Could you check a few things on this model? Use its own coordinates, in mm. Round coordinates to 2 decimals unless told otherwise and drop trailing zeros. Order: outer loops, then holes, each group sorted by start corner. A loop starts at its lowest first (then second) coordinate and runs counter-clockwise, first axis right, second up.
```python
from build123d import *

# Parameters (mm, degrees)
SKETCH1_W                                = 73
SKETCH1_H                                = 48
BOSS_EXTRUDE1_DEPTH                      = 1.6
CUT_EXTRUDE1_DEPTH                       = 44.712812767
MIRROR1_AT_THE_SECOND_PLANE_COPY_1_DEPTH = 44.712812767
FILLET1_R                                = 2
SKETCH3_R                                = 1.5
CUT_EXTRUDE2_DEPTH                       = 44.712812767


with BuildPart() as part:
    # Sketch1 → Boss-Extrude1 (new body)
    with BuildSketch(Plane.XY):
        Rectangle(SKETCH1_W, SKETCH1_H)
    extrude(amount=BOSS_EXTRUDE1_DEPTH)

    # Sketch2 → Cut-Extrude1 (cut, through all)
    with BuildSketch(Plane.XY.offset(1.6)):
        with BuildLine():
            Line((-27.5, 23), (-27.5, 24))
            Line((-27.5, 24), (-36.5, 24))
            Line((-36.5, 24), (-36.5, 15))
            Line((-36.5, 15), (-35.5, 15))
            ThreePointArc((-35.5, 15), (-29.843145751, 17.343145751), (-27.5, 23))
        make_face()
    cut_extrude1 = extrude(amount=-CUT_EXTRUDE1_DEPTH, mode=Mode.SUBTRACT)

    # Mirror1: Cut-Extrude1 across plane
    add(cut_extrude1.mirror(Plane(origin=(0, 0, 0), x_dir=(0, 0, 1), z_dir=(1, 0, 0))), mode=Mode.SUBTRACT)

    # Mirror1 at the second plane: Cut-Extrude1 across plane
    add(cut_extrude1.mirror(Plane.ZX), mode=Mode.SUBTRACT)

    # Mirror1 at the second plane copy 1 sketc → Mirror1 at the second plane copy 1 (cut, through all)
    with BuildSketch(Plane(origin=(0, 0, 1.6), x_dir=(-1, 0, 0), z_dir=(0, 0, 1))):
        with BuildLine():
            Line((-27.5, 23), (-27.5, 24))
            Line((-27.5, 24), (-36.5, 24))
            Line((-36.5, 24), (-36.5, 15))
            Line((-36.5, 15), (-35.5, 15))
            ThreePointArc((-35.5, 15), (-29.843145751, 17.343145751), (-27.5, 23))
        make_face()
    extrude(amount=-MIRROR1_AT_THE_SECOND_PLANE_COPY_1_DEPTH, mode=Mode.SUBTRACT)

    # Fillet1
    # the kernel refuses this fillet: 2 mm, written as the material it takes off along each edge
    with BuildSketch(Plane(origin=(-36.5, 15, 6.474685928), x_dir=(0.9997519364152339, 0.022272530929157337, 0), z_dir=(0, 0, -1)), Plane(origin=(-27.5, -24, 6.474685928), x_dir=(-0.022272530929167148, 0.9997519364152335, 0), z_dir=(0, 0, -1)), Plane(origin=(36.5, -15, 6.474685928), x_dir=(-0.9997519364152339, -0.022272530929157337, 0), z_dir=(0, 0, -1))) as fillet1_piece_1:
        with BuildLine():
            CenterArc((1.956075236, 1.99393574), FILLET1_R, 181.276227552, 84.260829523)
            Line((-0.043428637, 1.949390678), (-0.243379025, 1.944936172))
            Line((-0.243379025, 1.944936172), (-0.199950387, -0.004454506))
            Line((-0.199950387, -0.004454506), (0.004454506, -0.199950387))
            ThreePointArc((0.004454506, -0.199950387), (1.004206443, -0.177677856), (1.784883764, -0.199393574))
            Line((1.784883764, -0.199393574), (1.800446625, 0))
        make_face()
    extrude(amount=11.349371855, mode=Mode.SUBTRACT)
    with BuildSketch(Plane(origin=(-27.5, 24, 6.474685928), x_dir=(1, 0, 0), z_dir=(0, 0, -1)), Plane(origin=(-36.5, -15, 6.474685928), x_dir=(0, 1, 0), z_dir=(0, 0, -1)), Plane(origin=(36.5, 15, 6.474685928), x_dir=(0, -1, 0), z_dir=(0, 0, -1)), Plane(origin=(27.5, -24, 6.474685928), x_dir=(-1, 0, 0), z_dir=(0, 0, -1))) as fillet1_piece_2:
        with BuildLine():
            CenterArc((1.949874371, 2), FILLET1_R, 185.739170477, 84.260829523)
            Line((-0.040100503, 1.8), (-0.239097991, 1.78))
            ThreePointArc((-0.239097991, 1.78), (-0.2, 1), (-0.2, 0))
            Line((-0.2, 0), (0, -0.2))
            Line((0, -0.2), (1.949874371, -0.2))
            Line((1.949874371, -0.2), (1.949874371, 0))
        make_face()
    extrude(amount=11.349371855, mode=Mode.SUBTRACT)
    with BuildSketch(Plane(origin=(27.5, 24, 6.474685928), x_dir=(-1, 0, 0), z_dir=(0, 0, -1))) as fillet1_piece_3:
        with BuildLine():
            CenterArc((1.949874371, -2), FILLET1_R, 90, 84.260829523)
            Line((-0.040100503, -1.8), (-0.239097991, -1.78))
            ThreePointArc((-0.239097991, -1.78), (-0.2, -1), (-0.2, 0))
            Line((-0.2, 0), (0, 0.2))
            Line((0, 0.2), (1.949874371, 0.2))
            Line((1.949874371, 0.2), (1.949874371, 0))
        make_face()
    extrude(amount=11.349371855, mode=Mode.SUBTRACT)

    # Sketch3 → Cut-Extrude2 (cut, through all)
    with BuildSketch(Plane.XY.offset(1.6)):
        with Locations((-32, 0)):
            Circle(SKETCH3_R)
        with Locations((32, 0)):
            Circle(SKETCH3_R)
    extrude(amount=-CUT_EXTRUDE2_DEPTH, mode=Mode.SUBTRACT)


solid = part.part
```
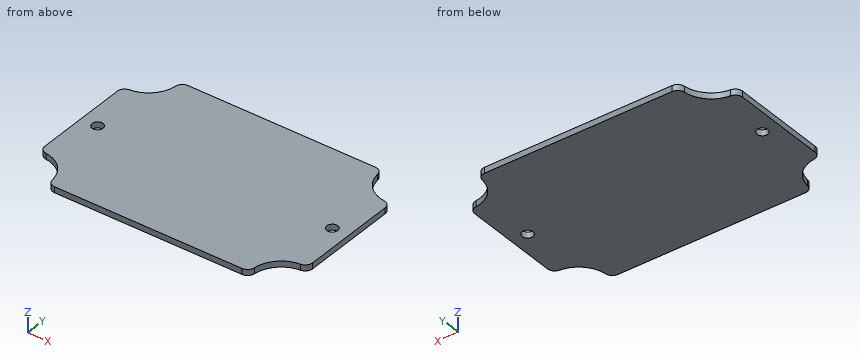
Q1. Imagine slicing it at B-B, the plane x = 32. Please give me the cut outline in (y, z), then the cut area to 3 significant figures.
Q2. Imagine slicing it at D-D, the plane y = -17.5. Please give me the cut outline in (x, z).
Q3. Imagine slicing it at C-C, the plane z = 0.25. Please give me the cut outline in (x, y), then the cut area to 3 significant figures.
Q4. Imagine slicing it at A-A, the plane y = 0. Please give me the cut outline in (x, z).
Q5. For P1, Ø4, axis at x = -32, y = 0, coming from the -Z side, with a flat end and sliding along its axis, tell me the tip position at first contact or that it passes through.
Q6. I need wall thicknesses on L1, parallel to X at y = 0.5, z = 0.5; L2, parallel to Y at x = -32, z = 0.6; L3, parallel to Y at x = -31.5, z = 1. Which ranges of each line are inside material? Lowest first, please.
Filled in:
1. outline: (-15.81, 0) - (-1.5, 0) - (-1.5, 1.6) - (-15.81, 1.6) - close; (1.5, 0) - (15.81, 0) - (15.81, 1.6) - (1.5, 1.6) - close
1. area: 45.8 mm2
2. outline: (-29.69, 0) - (29.69, 0) - (29.69, 1.6) - (-29.69, 1.6) - close
3. outline: (-36.5, -13.05) arc R2 ccw to (-34.7, -15.04) arc R8 cw to (-27.54, -22.2) arc R2 ccw to (-25.55, -24) - (25.55, -24) arc R2 ccw to (27.54, -22.2) arc R8 cw to (34.7, -15.04) arc R2 ccw to (36.5, -13.05) - (36.5, 13.05) arc R2 ccw to (34.7, 15.04) arc R8 cw to (27.54, 22.2) arc R2 ccw to (25.55, 24) - (-25.55, 24) arc R2 ccw to (-27.54, 22.2) arc R8 cw to (-34.7, 15.04) arc R2 ccw to (-36.5, 13.05) - close; hole circle Ø3 at (-32, 0); hole circle Ø3 at (32, 0)
3. area: 3,210 mm2
4. outline: (-36.5, 0) - (-33.5, 0) - (-33.5, 1.6) - (-36.5, 1.6) - close; (-30.5, 0) - (30.5, 0) - (30.5, 1.6) - (-30.5, 1.6) - close; (33.5, 0) - (36.5, 0) - (36.5, 1.6) - (33.5, 1.6) - close
5. P1: stops at z = 0
6. L1: x = -36.5 to -33.41, -30.59 to 30.59, 33.41 to 36.5
6. L2: y = -15.81 to -1.5, 1.5 to 15.81
6. L3: y = -16.07 to -1.41, 1.41 to 16.07
